Read the model definition and answer for the solid it produces. Units are mm, in the model's axes. Face numbers are marked on the shaded views. Coordinates: 2 decimals unless noted, no trailing zeros. Write each loop counter-clockwise with the first axis right and the second up, starting at its lowest first coordinate (ties: lowest second). Pieces come first, ordered by that corner, then holes. Notation, with made-up numbers: (55, 6) -> (87, 6) arc R13 cw to (87, 22) -> close; hole circle Ø9 at (56, 39). An arc over 180 degrees is marked (long way). Return JSON: item names as keys, results as strings.
from build123d import *

# Parameters (mm, degrees)
F0_W     = 188
F0_H     = 67
F1_DEPTH = 2.4
F2_R     = 2.8
F3_DEPTH = 5
F2_W     = 10
F2_H     = 10
F4_DEPTH = 10
F2_W_2   = 2.5
F2_H_2   = 7
F2_W_3   = 1.2939542532
F2_W_4   = 1.2059563398
F2_H_3   = 8.3965584815
F2_W_5   = 1.2060457468
F2_W_6   = 1.2940436602
F5_DEPTH = 25
F2_W_7   = 30.5
F6_DEPTH = 3.8
F7_R     = 0.45
F8_DEPTH = 67.001


with BuildPart() as f1:
    # F0 (on Top) → F1 (new body)
    with BuildSketch(Plane.XY):
        Rectangle(F0_W, F0_H)
    extrude(amount=F1_DEPTH)

    # F2 (on face) → F3 (join)
    with BuildSketch(Plane(origin=(0, 0, 0), x_dir=(1, 0, 0), z_dir=(0, 0, -1))):
        with Locations((66, 24.5)):
            Circle(F2_R)
        with Locations((33, 24.5)):
            Circle(F2_R)
        with Locations((0, 24.5)):
            Circle(F2_R)
        with Locations((-33, 24.5)):
            Circle(F2_R)
        with Locations((-66, 24.5)):
            Circle(F2_R)
    extrude(amount=F3_DEPTH)

    # F2 (on face) → F4 (join)
    with BuildSketch(Plane(origin=(0, 0, 0), x_dir=(1, 0, 0), z_dir=(0, 0, -1))):
        with Locations((89, -28.5)):
            Rectangle(F2_W, F2_H)
        with Locations((89, 28.5)):
            Rectangle(F2_W, F2_H)
        with Locations((-89, -28.5)):
            Rectangle(F2_W, F2_H)
        with Locations((-89, 28.5)):
            Rectangle(F2_W, F2_H)
    extrude(amount=F4_DEPTH)

    # F2 (on face) → F5 (join)
    with BuildSketch(Plane(origin=(0, 0, 0), x_dir=(1, 0, 0), z_dir=(0, 0, -1))):
        with Locations((-49.5, -6.8)):
            Rectangle(F2_W_2, F2_H_2)
        with Locations((-16.5, -6.8)):
            Rectangle(F2_W_2, F2_H_2)
        with Locations((16.5, -6.8)):
            Rectangle(F2_W_2, F2_H_2)
        with Locations((49.5, -6.8)):
            Rectangle(F2_W_2, F2_H_2)
        with Locations((-81.8969771266, -6.8)):
            Rectangle(F2_W_3, F2_H_2)
        with Locations((83.1470218301, -6.8)):
            Rectangle(F2_W_4, F2_H_2)
        Polygon((-82.5439542532, -3.3), (-81.25, -3.3), (-81.25, 5.0965584815), (-83.75, 5.0965584815), (-83.75, -3.3), align=None)
        with Locations((-49.5, 0.8982792407)):
            Rectangle(F2_W_2, F2_H_3)
        with Locations((-16.5, 0.8982792407)):
            Rectangle(F2_W_2, F2_H_3)
        with Locations((16.5, 0.8982792407)):
            Rectangle(F2_W_2, F2_H_3)
        with Locations((49.5, 0.8982792407)):
            Rectangle(F2_W_2, F2_H_3)
        Polygon((82.5440436602, -3.3), (83.75, -3.3), (83.75, 5.0965584815), (81.25, 5.0965584815), (81.25, -3.3), align=None)
        with Locations((-83.1469771266, -6.8)):
            Rectangle(F2_W_5, F2_H_2)
        with Locations((81.8970218301, -6.8)):
            Rectangle(F2_W_6, F2_H_2)
    extrude(amount=F5_DEPTH)

    # F2 (on face) → F6 (join)
    with BuildSketch(Plane(origin=(0, 0, 0), x_dir=(1, 0, 0), z_dir=(0, 0, -1))):
        with Locations((66, -6.8)):
            Rectangle(F2_W_7, F2_H_2)
        with Locations((33, -6.8)):
            Rectangle(F2_W_7, F2_H_2)
        with Locations((0, -6.8)):
            Rectangle(F2_W_7, F2_H_2)
        with Locations((-33, -6.8)):
            Rectangle(F2_W_7, F2_H_2)
        with Locations((-66, -6.8)):
            Rectangle(F2_W_7, F2_H_2)
    extrude(amount=F6_DEPTH)

    # F7 (on face) → F8 (cut, through all)
    with BuildSketch(Plane(origin=(0, 33.5, 0), x_dir=(-1, 0, 0), z_dir=(0, 1, 0))):
        with Locations((89, -5)):
            Circle(F7_R)
        with Locations((-89, -5)):
            Circle(F7_R)
    extrude(amount=-F8_DEPTH, mode=Mode.SUBTRACT)


solid = f1.part
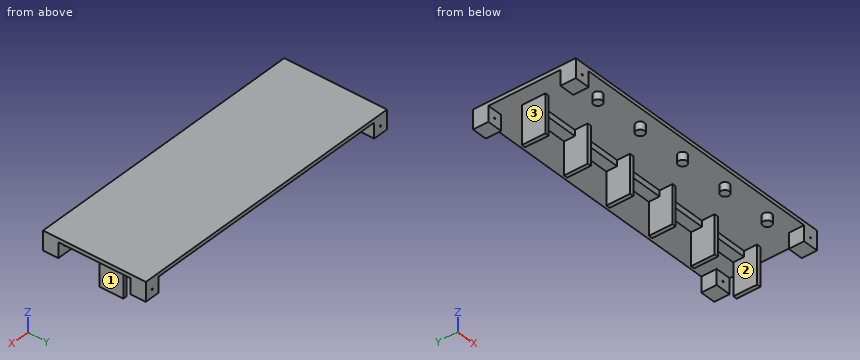
1. The part is cut by section C-C (y = 8). Determine the outline of the cut face in (x, z), then the cut area to 3 significant figures.
Taken from the geometry:
{"outline": "(-94, 0) -> (-83.75, 0) -> (-83.75, -25) -> (-81.25, -25) -> (-81.25, -3.8) -> (-50.75, -3.8) -> (-50.75, -25) -> (-48.25, -25) -> (-48.25, -3.8) -> (-17.75, -3.8) -> (-17.75, -25) -> (-15.25, -25) -> (-15.25, -3.8) -> (15.25, -3.8) -> (15.25, -25) -> (17.75, -25) -> (17.75, -3.8) -> (48.25, -3.8) -> (48.25, -25) -> (50.75, -25) -> (50.75, -3.8) -> (81.25, -3.8) -> (81.25, -25) -> (83.75, -25) -> (83.75, 0) -> (94, 0) -> (94, 2.4) -> (-94, 2.4) -> close", "area": "1,410 mm2"}
2. The part is cut by section A-A (z = -20.5). Determine the outline of the cut face in (x, y).
Taken from the geometry:
{"outline": "(-83.75, -5.1) -> (-81.25, -5.1) -> (-81.25, 10.3) -> (-83.75, 10.3) -> close; (-50.75, -5.1) -> (-48.25, -5.1) -> (-48.25, 10.3) -> (-50.75, 10.3) -> close; (-17.75, -5.1) -> (-15.25, -5.1) -> (-15.25, 10.3) -> (-17.75, 10.3) -> close; (15.25, -5.1) -> (17.75, -5.1) -> (17.75, 10.3) -> (15.25, 10.3) -> close; (48.25, -5.1) -> (50.75, -5.1) -> (50.75, 10.3) -> (48.25, 10.3) -> close; (81.25, -5.1) -> (83.75, -5.1) -> (83.75, 10.3) -> (81.25, 10.3) -> close"}
3. For a pull along X with two mould halves and no side action, classify the marked faces 1, 2 and 3 as +X half, -X half, draft (parallel to the pull), parting line (faces both ways), or undercut.
Taken from the geometry:
{"face 1": "+X half", "face 2": "undercut", "face 3": "-X half"}
4. Consider L1, parallel to X at y = -3, z = -15.75; L2, parallel to Y at x = -66, z = -1.5; L3, parallel to Z at x = -89, y = -29.25. Determine where each line is inside the solid, lowest interval first.
Taken from the geometry:
{"L1": "x = -83.75 to -81.25, -50.75 to -48.25, -17.75 to -15.25, 15.25 to 17.75, 48.25 to 50.75, 81.25 to 83.75", "L2": "y = -27.3 to -21.7, 3.3 to 10.3", "L3": "z = -10 to -5.45, -4.55 to 2.4"}
5. The part is cut by section B-B (x = -73). Determine the outline of the cut face in (y, z), then the cut area to 3 significant figures.
Taken from the geometry:
{"outline": "(-33.5, 0) -> (3.3, 0) -> (3.3, -3.8) -> (10.3, -3.8) -> (10.3, 0) -> (33.5, 0) -> (33.5, 2.4) -> (-33.5, 2.4) -> close", "area": "187 mm2"}
6. Flat-ended cylindrical pins translate along their axes: pin 1 Ø11 at (x, y) = (89, -26.5) entering from -Z; pin 2 Ø12.5 at (y, z) = (2, -11.5) entering from -X; pin 3 Ø5 at (y, z) = (-7, -7) entering from +X; pin 4 Ø1 at (y, z) = (-25, -11.5) entering from +X. Find the tip coordinate at first contact, or state that the pin passes through.
Taken from the geometry:
{"pin 1": "stops at z = -10", "pin 2": "stops at x = -83.75", "pin 3": "stops at x = 83.75", "pin 4": "passes through"}
7. The part is cut by section D-D (x = 0). Determine the outline of the cut face in (y, z).
Taken from the geometry:
{"outline": "(-33.5, 0) -> (-27.3, 0) -> (-27.3, -5) -> (-21.7, -5) -> (-21.7, 0) -> (3.3, 0) -> (3.3, -3.8) -> (10.3, -3.8) -> (10.3, 0) -> (33.5, 0) -> (33.5, 2.4) -> (-33.5, 2.4) -> close"}
